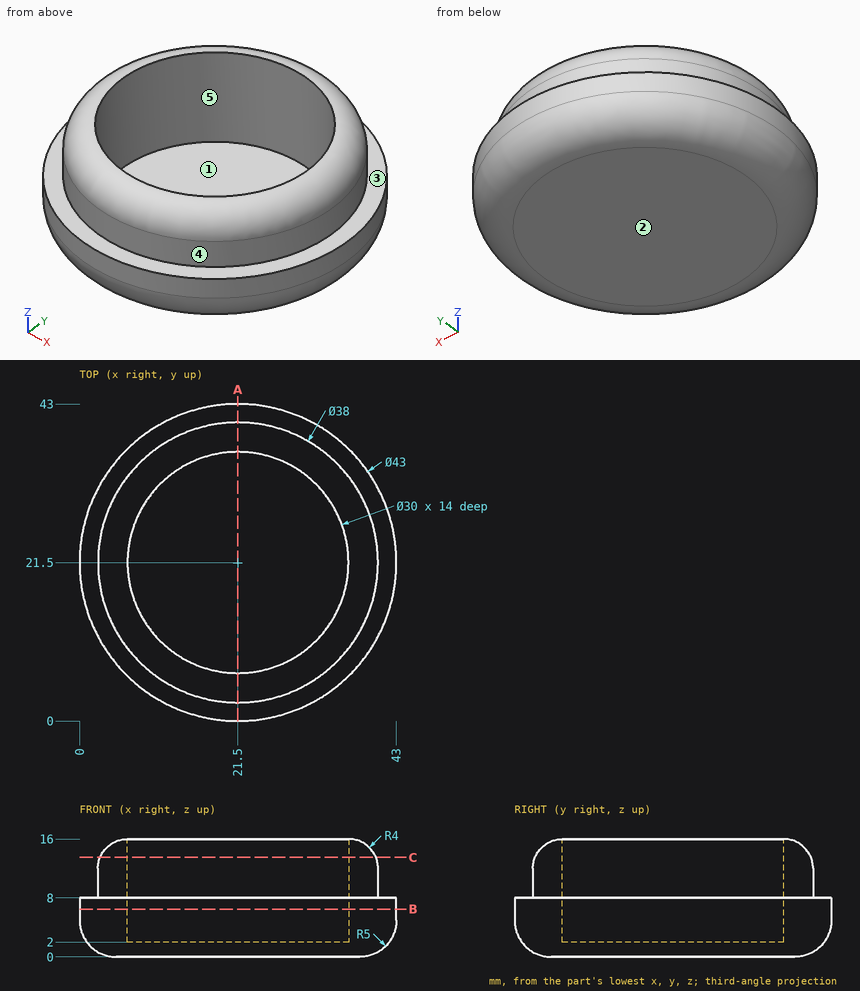
Source: three-view drawing plus pictorial views. Frame: mm from the lowest corner of the part. A direction names the side the tool comes from. Give positions to 0.01 mm unless a question says otherwise; leave off trailing zeros. Loops run counter-clockwise (first coordinate to the right, second up) from the corner with the lowest first, then second, coordinate; pieces in that order, holes last. Notation, with made-up numbers: M 41,16.25 L 52,16.25 A25 cw 52,34.25 Z; hole C -19,53.25 d7. An arc over 180 degrees is marked long. Put each result on its own line as item: value.
Q1. Section B-B (z = 6.5). Return the cut outline in (x, y).
Response values:
outline: C 21.5,21.5 d43; hole C 21.5,21.5 d30
Q2. Mould query, pull axis Y, two halves, no side actions, for the marked faces 3, 4 and 5. Classes: released by +Y, released by -Y, zero draft, split by the parting line, or undercut.
Response values:
face 3: zero draft
face 4: split by the parting line
face 5: undercut
Q3. Line query: probe 1 along Y at (x, z) = (21.5, 9); probe 2 along Z at (x, y) = (16, 23.5); probe 3 along Y at (x, z) = (21.5, 6). Output: solid intervals per line, ascending. Write a range as [from, to].
Response values:
probe 1: y = [2.5, 6.5], [36.5, 40.5]
probe 2: z = [0, 2]
probe 3: y = [0, 6.5], [36.5, 43]
Q4. Reachability of the marked faces 1 and 2 from +Z, -Z, +X, -X, +Y, -Y: full face, straight path, thin tool, end or side. Return the list, or none.
Response values:
face 1: +Z
face 2: -Z, +X, -X, +Y, -Y
Q5. Pin query (flat end, axial travel): P1, Ø8, axis at y = 28.5, z = 13.5, coming from the +X side; P2, Ø4, axis at y = 35.5, z = 4.5, coming from the +X side; P3, Ø2, axis at x = 13.5, y = 37.5, coming from the -Z side. Return the tip coordinate at first contact, or that it passes through.
Response values:
P1: stops at x = 40.22
P2: stops at x = 39.32
P3: stops at z = 0.02
Q6. Section C-C (z = 13.5). Return the cut outline in (x, y).
Response values:
outline: C 21.5,21.5 d37.42; hole C 21.5,21.5 d30
Q7. Section A-A (x = 21.5). Return the cut outline in (y, z), and give its area (3 significant figures).
Response values:
outline: M 0,5 A5 ccw 5,0 L 38,0 A5 ccw 43,5 L 43,8 L 40.5,8 L 40.5,12 A4 ccw 36.5,16 L 36.5,2 L 6.5,2 L 6.5,16 A4 ccw 2.5,12 L 2.5,8 L 0,8 Z
area: 210 mm²
